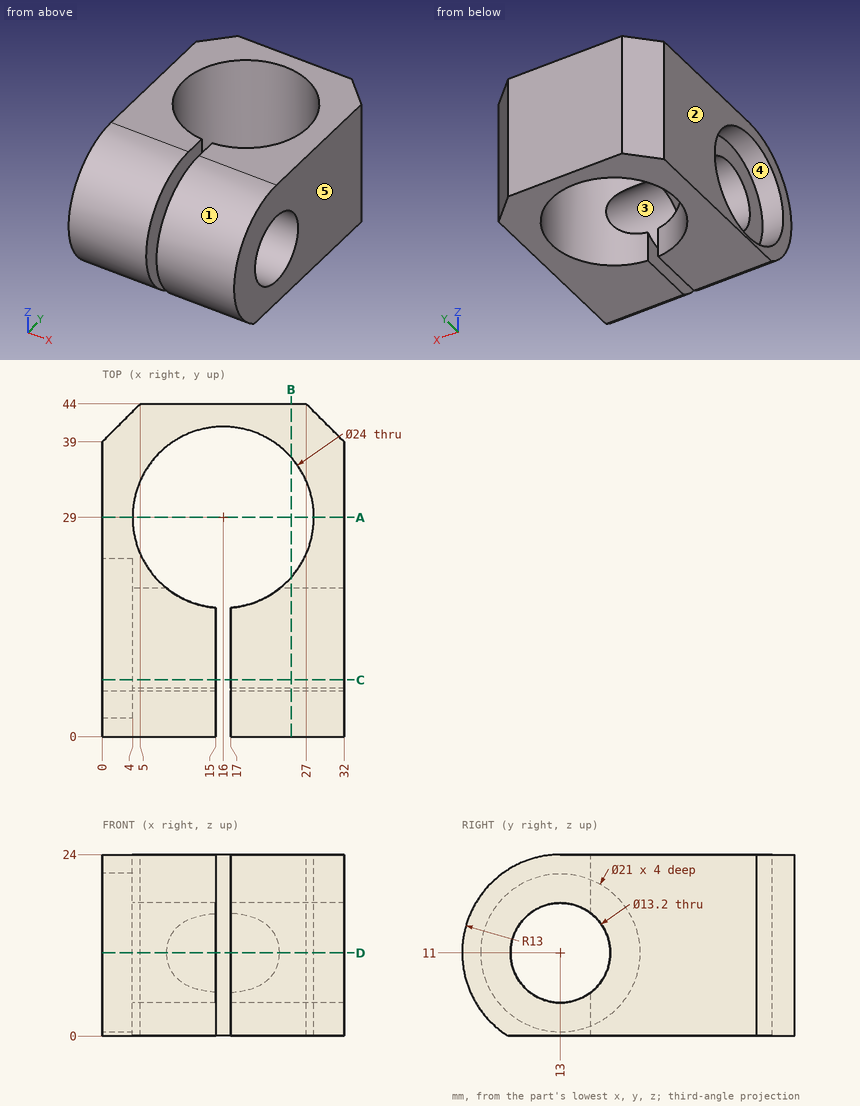
Job drawing, mm, ordinate dimensions from the low corner. One solid piece. A direction names the side the tool comes from. Round coordinates to 2 decimals unless told otherwise and drop trailing zeros. Write each loop counter-clockwise with the first axis right and the second up, starting at its lowest first coordinate (ties: lowest second). Pieces come first, ordered by that corner, then holes. Notation, with made-up numbers: M 51.5,83.5 L 105.5,83.5 A11 cw 105.5,102.5 Z; hole C -23,86.5 d9. An arc over 180 degrees is marked long. Return JSON: item names as keys, results as strings. Group by question number.
(1) Saw through at B-B on x = 25. Write the cut outline in (y, z).
(2) Saw through at D-D on z = 11. Write the cut outline in (x, y), then the cut area to 3 significant figures.
(3) Which spindle directions (+Z, -Z, +X, -X, +Y, -Y) get a long thin tool onto all of the face, cutting with end or side? Do the marked faces 4 and 5. Say none if no direction does.
(4) Drill centre lines: probe 1 along X at (y, z) = (15, 22.5); probe 2 along Z at (x, y) = (20, 13); probe 3 along X at (y, z) = (29, 11). Where is each one in solid material? Low to high.
(5) Saw through at A-A on y = 29. Write the cut outline in (x, z), then the cut area to 3 significant figures.
(6) Two-plate mould, pull along Y, no slides. Class the marked faces 1, 2 and 3: +Y half, -Y half, draft (parallel to the pull), parting line (faces both ways), or undercut.
(7) Saw through at C-C on y = 7.5. Write the cut outline in (x, z).
(8) Pin check, flat tips, straight feed: pin 1 Ø1 at (y, z) = (18.5, 16) entering from -X; pin 2 Ø10 at (x, z) = (20, 18) entering from -Y; pin 3 Ø4 at (x, z) = (20.5, 8) entering from -Y. Stop position of each tip, or through.
Returned:
{
 "1": {"outline": "M 6.07,0 L 21.06,0 L 21.06,24 L 13,24 A13 ccw Z; M 36.94,0 L 44,0 L 44,24 L 36.94,24 Z; hole C 13,11 d13.2"},
 "2": {"outline": "M 0,0 L 15,0 L 15,6.4 L 4,6.4 L 4,2.5 L 0,2.5 Z; M 0,23.5 L 4,23.5 L 4,19.6 L 8.54,19.6 A12 cw long 23.46,19.6 L 32,19.6 L 32,39 L 27,44 L 5,44 L 0,39 Z; M 17,0 L 32,0 L 32,6.4 L 17,6.4 Z", "area": "491 mm²"},
 "3": {"face 4": "-X", "face 5": "+Z, -Z, +X, +Y, -Y"},
 "4": {"probe 1": "0 to 15, 17 to 32", "probe 2": "0 to 4.4, 17.6 to 24", "probe 3": "0 to 4, 28 to 32"},
 "5": {"outline": "M 0,0 L 4,0 L 4,24 L 0,24 Z; M 28,0 L 32,0 L 32,24 L 28,24 Z", "area": "192 mm²"},
 "6": {"face 1": "-Y half", "face 2": "draft", "face 3": "undercut"},
 "7": {"outline": "M 0,0 L 15,0 L 15,7.35 L 4,7.35 L 4,2.06 L 0,2.06 Z; M 0,19.94 L 4,19.94 L 4,14.65 L 15,14.65 L 15,22.78 L 0,22.78 Z; M 17,0 L 32,0 L 32,7.35 L 17,7.35 Z; M 17,14.65 L 32,14.65 L 32,22.78 L 17,22.78 Z"},
 "8": {"pin 1": "x = 4", "pin 2": "y = 0.15", "pin 3": "y = 0.04"}
}
